For this review, take the finished solid that the model builds, in its own axes (mm). A direction names the side the tool comes from. Give positions to 0.01 mm unless a question says otherwise; leave off trailing zeros. Order: outer loops, then holes, each group sorted by start corner. A loop starts at its lowest first (then second) coordinate and runs counter-clockwise, first axis right, second up.
Item 1: For probe 1 along X at (y, z) = (26.5, 6); probe 2 along Z at (x, y) = (30, 2), list the stretches that pass through material, from the lowest coordinate up.
Item 2: For P1, Ø12, axis at x = 5.5, z = 10.5, coming from the +Y side; P2, Ø0.6, axis at y = 29.5, z = 0.5, coming from the +X side; P3, Ø1, axis at y = 10, z = 1.5, coming from the +X side; P4, Ø8, axis at x = 33.5, z = 9, coming from the +Y side, all flat-tipped, find the tip position at first contact; note any pin that passes through.
Item 3: Machinability: for faces 1 (the flat face through (40, 7, 1)), 2 (the flat face through (2, 3, 20)), 3 (the flat face through (0, 25, 11)), which of the approach directions +Z, -Z, +X, -X, +Y, -Y give a long, thin tool a straight path to every point of the face, cutting with its end or side? Answer none if there is none.
Item 4: Consider section A-A (z = 9). Give the boundary of the cut face in (x, y), plus the area to 3 significant figures.
Item 5: Consider section C-C (y = 14). Give the boundary of the cut face in (x, z).
Item 6: Consider section D-D (z = 17.25). Give the boundary of the cut face in (x, y), plus the area to 3 significant figures.
Item 7: Consider section B-B (x = 26). Give the boundary of the cut face in (y, z).
```python
from build123d import *

# Parameters (mm, degrees)
F1_DEPTH = 2
F3_DEPTH = 20
F4_R     = 10


with BuildPart() as f1:
    # F0 (on Top) → F1 (new body)
    with BuildSketch(Plane.XY):
        Polygon((15, 40), (0, 40), (0, 0), (40, 0), (40, 15), (15, 15), align=None)
    extrude(amount=F1_DEPTH)

    # F2 (on Top) → F3 (join)
    with BuildSketch(Plane.XY):
        Polygon((0, 0), (0, 40), (-2, 40), (-2, -2), (40.175851, -2), (40.175851, 0), align=None)
    extrude(amount=F3_DEPTH)

    # F4
    f4_edges = [f1.edges().sort_by_distance(p)[0] for p in [
        (0, 0, 11),
        (15, 15, 1),
        (-2, -2, 10),
        (-1, 40, 20),
        (40.175851, -1, 20),
    ]]
    fillet(f4_edges, radius=F4_R)


solid = f1.part
```
Resolved:
1. probe 1: x = -2 to 0
1. probe 2: z = 0 to 2
2. P1: stops at y = 40
2. P2: stops at x = 15
2. P3: stops at x = 40
2. P4: stops at y = 0
3. face 1: +Z, -Z, +X, +Y
3. face 2: +Z, +X, -X, +Y, -Y
3. face 3: +Z, +X, +Y
4. outline: (-2, 8) arc R10 ccw to (8, -2) - (40.18, -2) - (40.18, 0) - (10, 0) arc R10 cw to (0, 10) - (0, 40) - (-2, 40) - close
4. area: 164 mm2
5. outline: (-2, 0) - (40, 0) - (40, 2) - (0, 2) - (0, 20) - (-2, 20) - close
6. outline: (-2, 8) arc R10 ccw to (8, -2) - (37.06, -2) - (37.06, 0) - (10, 0) arc R10 cw to (0, 10) - (0, 36.89) - (-2, 36.89) - close
6. area: 152 mm2
7. outline: (-2, 0) - (15, 0) - (15, 2) - (0, 2) - (0, 20) - (-2, 20) - close
